from build123d import *

# Parameters (mm, degrees)
SKETCH_1_W           = 100
SKETCH_1_H           = 30
EXTRUDE_1_DEPTH      = 3
CUT_EXTRUDE_1_REACH  = 106.446
EXTRUDE_3_DEPTH      = 3
CUT_EXTRUDE_2_REACH  = 106.446
SKETCH_5_R           = 1.65
SKETCH_5_R_2         = 1.683787266
EXTRUDE_4_DEPTH      = 34
EXTRUDE_4_DEPTH_BACK = 3
SKETCH_6_W           = 3
SKETCH_6_H           = 30
EXTRUDE_5_DEPTH      = 30
CHAMFER_1_SIZE       = 3
CHAMFER_2_SIZE       = 3
EXTRUDE_6_DEPTH      = 3
CUT_EXTRUDE_3_DEPTH  = 114.481275989


with BuildPart() as part:
    # 草图1 → 凸台-拉伸1 (new body)
    with BuildSketch(Plane.XY):
        with Locations((50, 15)):
            Rectangle(SKETCH_1_W, SKETCH_1_H)
    extrude(amount=EXTRUDE_1_DEPTH)

    # 草图2 → 切除-拉伸1 (cut, up to next)
    with BuildSketch(Plane.XY.offset(3), mode=Mode.PRIVATE) as cut_extrude_1_sk1:
        Polygon((0, 18), (12, 30), (0, 30), align=None)
    cut_extrude_1_tool1 = extrude(cut_extrude_1_sk1.sketch, amount=-CUT_EXTRUDE_1_REACH, mode=Mode.PRIVATE) & part.part
    add(cut_extrude_1_tool1.solids().sort_by_distance((4, 26, 3))[0], mode=Mode.SUBTRACT)

    # 草图4 → 凸台-拉伸3 (add)
    with BuildSketch(Plane(origin=(0, 0, 0), x_dir=(-1, 0, 0), z_dir=(0, 0, -1))):
        Polygon((0, 0), (17, 0), (17, 1), (0, 18), align=None)
    extrude(amount=-EXTRUDE_3_DEPTH)

    # 草图5 → 切除-拉伸2 (cut, up to next)
    with BuildSketch(Plane.XY.offset(3), mode=Mode.PRIVATE) as cut_extrude_2_sk1:
        with Locations((9.963410089, 21.593670707)):
            Circle(SKETCH_5_R)
    cut_extrude_2_tool1 = extrude(cut_extrude_2_sk1.sketch, amount=-CUT_EXTRUDE_2_REACH, mode=Mode.PRIVATE) & part.part
    # 草图5 → 切除-拉伸2 (cut, up to next)
    with BuildSketch(Plane.XY.offset(3), mode=Mode.PRIVATE) as cut_extrude_2_sk2:
        with Locations((97, 26)):
            Circle(SKETCH_5_R_2)
    cut_extrude_2_tool2 = extrude(cut_extrude_2_sk2.sketch, amount=-CUT_EXTRUDE_2_REACH, mode=Mode.PRIVATE) & part.part
    # 草图5 → 切除-拉伸2 (cut, up to next)
    with BuildSketch(Plane.XY.offset(3), mode=Mode.PRIVATE) as cut_extrude_2_sk3:
        with Locations((97, 4)):
            Circle(SKETCH_5_R)
    cut_extrude_2_tool3 = extrude(cut_extrude_2_sk3.sketch, amount=-CUT_EXTRUDE_2_REACH, mode=Mode.PRIVATE) & part.part
    add(cut_extrude_2_tool1.solids().sort_by_distance((9.96341, 21.593671, 3))[0], mode=Mode.SUBTRACT)
    add(cut_extrude_2_tool2.solids().sort_by_distance((97, 26, 3))[0], mode=Mode.SUBTRACT)
    add(cut_extrude_2_tool3.solids().sort_by_distance((97, 4, 3))[0], mode=Mode.SUBTRACT)

    # 草图6 → 凸台-拉伸4 (add, two sides: drawn at the far end of the back side and taken through both)
    with BuildSketch(Plane.XY.offset(3).offset(-EXTRUDE_4_DEPTH_BACK)):
        with Locations((101.5, 15)):
            Rectangle(SKETCH_6_W, SKETCH_6_H)
    extrude(amount=EXTRUDE_4_DEPTH + EXTRUDE_4_DEPTH_BACK)

    # 草图7 → 凸台-拉伸5 (add)
    with BuildSketch(Plane.XY.offset(3)):
        Polygon((-17, 1), (12, 30), (12, 27.171572875), (-14.171572875, 1), (-14.171572875, 0), (-17, 0), align=None)
    extrude(amount=EXTRUDE_5_DEPTH)

    # 倒角1
    chamfer_1_edges = [part.edges().sort_by_distance(p)[0] for p in [
        (103, 15, 0),
    ]]
    chamfer(chamfer_1_edges, length=CHAMFER_1_SIZE)

    # 倒角2
    chamfer_2_edges = [part.edges().sort_by_distance(p)[0] for p in [
        (103, 15, 37),
    ]]
    chamfer(chamfer_2_edges, length=CHAMFER_2_SIZE - 0.0001)  # a hair under: the kernel refuses the full size

    # 草图3 → 凸台-拉伸6 (add)
    with BuildSketch(Plane(origin=(0, 0, 0), x_dir=(-1, 0, 0), z_dir=(0, 0, -1))):
        Polygon((-24, 0), (-10, -14), (-10, 0), align=None)
    extrude(amount=-EXTRUDE_6_DEPTH)

    # 草图8 → 切除-拉伸3 (cut, through all)
    with BuildSketch(Plane(origin=(0, 0, 0), x_dir=(-1, 0, 0), z_dir=(0, 0, -1))):
        with BuildLine():
            Line((-78.021683781, 21.894650921), (-78.021683781, 8.105349079))
            ThreePointArc((-78.021683781, 8.105349079), (-83.534405897, 2.592626964), (-89.047128012, 8.105349079))
            Line((-89.047128012, 8.105349079), (-89.047128012, 21.894650921))
            ThreePointArc((-89.047128012, 21.894650921), (-83.534405897, 27.407373036), (-78.021683781, 21.894650921))
        make_face()
        with BuildLine():
            Line((-53.021683781, 21.894650921), (-53.021683781, 8.105349079))
            ThreePointArc((-53.021683781, 8.105349079), (-58.534405897, 2.592626964), (-64.047128012, 8.105349079))
            Line((-64.047128012, 8.105349079), (-64.047128012, 21.894650921))
            ThreePointArc((-64.047128012, 21.894650921), (-58.534405897, 27.407373036), (-53.021683781, 21.894650921))
        make_face()
        with BuildLine():
            Line((-28.021683781, 21.894650921), (-28.021683781, 8.105349079))
            ThreePointArc((-28.021683781, 8.105349079), (-33.534405897, 2.592626964), (-39.047128012, 8.105349079))
            Line((-39.047128012, 8.105349079), (-39.047128012, 21.894650921))
            ThreePointArc((-39.047128012, 21.894650921), (-33.534405897, 27.407373036), (-28.021683781, 21.894650921))
        make_face()
    extrude(amount=-CUT_EXTRUDE_3_DEPTH, mode=Mode.SUBTRACT)


solid = part.part
Can you work these out from the model? Positions are in its coordinate system, mm. A direction names the side the tool comes from. Round coordinates to 2 decimals unless told otherwise and drop trailing zeros. Order: outer loops, then holes, each group sorted by start corner. A loop starts at its lowest first (then second) coordinate and runs counter-clockwise, first axis right, second up. Notation, with made-up numbers: M 45.25,5.25 L 49.25,5.25 A15 ccw 49.25,9.25 Z; hole C -29.5,42 d3. An arc over 180 degrees is marked long. Use a Markdown table: item, result.
1) On a 3-axis mill with a long thin cutter (end or side, diameter ignored), from which of +Z, -Z, +X, -X, +Y, -Y can I reach the whole of each face in a straight line? I mean faces 4 (the face through (89.047, 15, 1)), 5 (the face through (44, 13, 3)), 6 (the face through (75, 0, 2)), 7 (the face through (-1, 15, 33)). Say none if no direction works.
Geometry says:
| item | result |
|---|---|
| face 4 | +Z, -Z |
| face 5 | +Z, -Y |
| face 6 | +Z, -Z, +X, -Y |
| face 7 | +Z, -X, +Y, -Y |
2) If I drill on line 1 along Y through (x, z) = (97, 1.9); line 2 along X through (y, z) = (1, 19); line 3 along Z through (x, y) = (65.5, 16), over which ranges is the centre line in solid material (lowest first)?
Geometry says:
| item | result |
|---|---|
| line 1 | y = 0 to 2.35, 5.65 to 24.32, 27.68 to 30 |
| line 2 | x = -17 to -14.17, 100 to 103 |
| line 3 | z = 0 to 3 |
3) If we mould it in two halves opening along Y, with no side actions, what happens to faces 1 (the face through (10, -7, 1)), 2 (the face through (17, -7, 1)), 3 (the face through (98.606, 26.506, 1.521))? For each: +Y half, -Y half, draft (parallel to the pull), parting line (faces both ways), or undercut.
Geometry says:
| item | result |
|---|---|
| face 1 | draft |
| face 2 | -Y half |
| face 3 | undercut |
4) Imagine slicing it at C-C (y = 18). Give the number of separate pieces and of enclosed holes in the cut face, then the cut area to 3 significant figures.
Geometry says:
| item | result |
|---|---|
| separate pieces | 4 |
| enclosed holes | 0 |
| area | 388 mm² |
5) Imagine slicing it at B-B (x = 97). List the corners of the cut face in (y, z) for me.
Geometry says:
| item | result |
|---|---|
| outline | M 0,0 L 2.35,0 L 2.35,3 L 0,3 Z; M 5.65,0 L 24.32,0 L 24.32,3 L 5.65,3 Z; M 27.68,0 L 30,0 L 30,3 L 27.68,3 Z |
6) Imagine slicing it at A-A (z = 13). List the corners of the cut face in (x, y) for me, then the cut area to 3 significant figures.
Geometry says:
| item | result |
|---|---|
| outline | M -17,0 L -14.17,0 L -14.17,1 L 12,27.17 L 12,30 L -17,1 Z; M 100,0 L 103,0 L 103,30 L 100,30 Z |
| area | 171 mm² |
7) I'm going to push flat-ended pins straight in: P1, Ø0.9, axis at y = 15, z = 1, coming from the -X side; P2, Ø4.5, axis at x = 97, y = 4, coming from the +Z side; P3, Ø0.9, axis at y = 16, z = 2, coming from the -X side. Where does each tip first touch, or does it pass through?
Geometry says:
| item | result |
|---|---|
| P1 | stops at x = -3.45 |
| P2 | stops at z = 3 |
| P3 | stops at x = -2.45 |
